from build123d import *

# Parameters (mm, degrees)
BASE_FLANGE2_DEPTH             = 1
EDGE_FLANGE1_STRIP_W           = 6
EDGE_FLANGE1_STRIP_H           = 1
EDGE_FLANGE1_STRIP_CUT_DEPTH   = 82.6
EDGE_FLANGE1_STRIP_2_W         = 6
EDGE_FLANGE1_STRIP_2_H         = 1
EDGE_FLANGE1_STRIP_CUT_2_DEPTH = 82.6
EDGE_FLANGE1_DEPTH             = 82.6
EDGE_FLANGE1_BEND_DEPTH        = 82.6
SKETCH16_W                     = 66.6
SKETCH16_H                     = 7
CUT_EXTRUDE1_DEPTH             = 138.553195479
FILLET1_R                      = 1
SKETCH17_R                     = 2
CUT_EXTRUDE2_DEPTH             = 138.553195479
FILLET2_R                      = 2.5


# Sheet-metal steps are written as plain solids
with BuildPart() as part:
    # Sketch1 → Base-Flange2 (new body)
    with BuildSketch(Plane(origin=(0, 0, 0), x_dir=(1, 0, 0), z_dir=(0, 1, 0))):
        Polygon((0, 0), (0, 82.6), (5, 82.6), (12.071067812, 89.671067812), (92.000932188, 89.671067812), (99.072, 82.6), (104.072, 82.6), (104.072, 0), (99.072, 0), (92.000932188, -7.071067812), (12.071067812, -7.071067812), (5, 0), align=None)
    extrude(amount=-BASE_FLANGE2_DEPTH)

    # Edge-Flange1 strip (across the edge) → Edge-Flange1 strip cut (cut)
    with BuildSketch(Plane(origin=(104.072, 0, 0), x_dir=(-1, 0, 0), z_dir=(0, 0, -1))):
        with Locations((-1, -0.5)):
            Rectangle(EDGE_FLANGE1_STRIP_W, EDGE_FLANGE1_STRIP_H)
    extrude(amount=EDGE_FLANGE1_STRIP_CUT_DEPTH, mode=Mode.SUBTRACT)

    # Edge-Flange1 strip 2 (across the edge) → Edge-Flange1 strip cut 2 (cut)
    with BuildSketch(Plane.XY.offset(-82.6)):
        with Locations((-1, -0.5)):
            Rectangle(EDGE_FLANGE1_STRIP_2_W, EDGE_FLANGE1_STRIP_2_H)
    extrude(amount=EDGE_FLANGE1_STRIP_CUT_2_DEPTH, mode=Mode.SUBTRACT)

    # Edge-Flange1 section (across the edge) → Edge-Flange1 (add)
    with BuildSketch(Plane(origin=(104.072, 0, 0), x_dir=(-1, 0, 0), z_dir=(0, 0, -1))):
        with BuildLine():
            Line((0, 1), (0, 7))
            Line((0, 7), (1, 7))
            Line((1, 7), (1, 1))
            ThreePointArc((1, 1), (1.292893219, 0.292893219), (2, 0))
            Line((2, 0), (2, -1))
            ThreePointArc((2, -1), (0.585786438, -0.414213562), (0, 1))
        make_face()
    extrude(amount=EDGE_FLANGE1_DEPTH)

    # Edge-Flange1 section 2 (across the edge) → Edge-Flange1 bend (add)
    with BuildSketch(Plane.XY.offset(-82.6)):
        with BuildLine():
            Line((0, 1), (0, 7))
            Line((0, 7), (1, 7))
            Line((1, 7), (1, 1))
            ThreePointArc((1, 1), (1.292893219, 0.292893219), (2, 0))
            Line((2, 0), (2, -1))
            ThreePointArc((2, -1), (0.585786438, -0.414213562), (0, 1))
        make_face()
    extrude(amount=EDGE_FLANGE1_BEND_DEPTH)

    # Sketch16 → Cut-Extrude1 (cut, through all)
    with BuildSketch(Plane(origin=(104.072, 0, 0), x_dir=(0, 0, -1), z_dir=(1, 0, 0))):
        with Locations((41.3, 4.5)):
            Rectangle(SKETCH16_W, SKETCH16_H)
    extrude(amount=-CUT_EXTRUDE1_DEPTH, mode=Mode.SUBTRACT)

    # Fillet1
    fillet1_edges = [part.edges().sort_by_distance(p)[0] for p in [
        (0.5, 7, -74.6),
        (0.5, 7, -8),
        (103.572, 7, -8),
        (103.572, 7, -74.6),
        (103.572, 7, 0),
        (103.572, 7, -82.6),
        (0.5, 7, -82.6),
        (0.5, 7, 0),
    ]]
    fillet(fillet1_edges, radius=FILLET1_R)

    # Sketch17 → Cut-Extrude2 (cut, through all)
    with BuildSketch(Plane(origin=(104.072, 0, 0), x_dir=(0, 0, -1), z_dir=(1, 0, 0))):
        with Locations(Location((4, 4, 0), (0, 0, 90))):
            Circle(SKETCH17_R)
        with Locations(Location((78.6, 4, 0), (0, 0, 90))):
            Circle(SKETCH17_R)
    extrude(amount=-CUT_EXTRUDE2_DEPTH, mode=Mode.SUBTRACT)

    # Fillet2
    fillet2_edges = [part.edges().sort_by_distance(p)[0] for p in [
        (12.071067812, -0.5, -89.671067812),
        (92.000932188, -0.5, -89.671067812),
        (92.000932188, -0.5, 7.071067812),
        (12.071067812, -0.5, 7.071067812),
    ]]
    fillet(fillet2_edges, radius=FILLET2_R)


solid = part.part
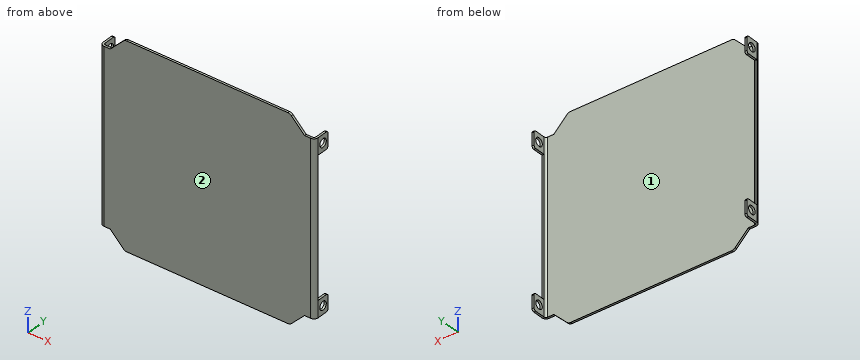
For this review, take the finished solid that the model builds, in its own axes (mm). Face numbers are marked on the shaded views. A direction names the side the tool comes from. Coordinates: 2 decimals unless noted, no trailing zeros. Write each loop counter-clockwise with the first axis right and the second up, starting at its lowest first coordinate (ties: lowest second). Pieces come first, ordered by that corner, then holes. Notation, with made-up numbers: (45.25, 5.5) -> (88.25, 5.5) arc R15 ccw to (88.25, 32.5) -> close; hole circle Ø8 at (-15.75, 79.5). An arc over 180 degrees is marked (long way). Write each question's results on one line, items separated by ' | '. Start each with the question number.
1) Wall thickness on L1, parallel to Z at x = 103.6, y = 4; L2, parallel to X at y = 3.75, z = -75.5; L3, parallel to Y at x = 99, z = -74.5: over which ranges is each line inside the solid? List them lowest first. Write a range as [from, to].
2) For the marked faces 1 and 2, list the 3-axis set-ups (+Z, -Z, +X, -X, +Y, -Y) from which the entire face can be reached by the end or side of a thin tool; tool diameter is ignored.
3) Consider section A-A (z = -4). Write out the cut boundary in (x, y), plus the area to 3 significant figures.
4) Consider section C-C (z = -42). Write out the cut boundary in (x, y).
5) Consider section B-B (y = 4). Give the number of separate pieces and of enclosed holes in the cut face, plus the area to 3 significant figures.
6) Consider section D-D (x = 74). Write out the cut boundary in (y, z).
7) Insertion check: pin 1 (0.8 mm diameter, centred on x = 0.5, z = -38, fed in from +Y); pin 2 (12 mm diameter, centred on x = 74.5, z = -27, fed in from +Y); pin 3 (0.5 mm diameter, centred on x = 0.5, y = 3.5, fed in from -Z); pin 4 (1.5 mm diameter, centred on x = 100.5, y = 1.5, fed in from +Z). Each pin has a flat end and moves straight along its axis. Give the tip position at first contact, or say it passes through.
Geometry says:
1) L1: [-82.6, -80.6], [-76.6, -74.6], [-8, -6], [-2, 0] | L2: [0, 1], [103.07, 104.07] | L3: [-1, 0]
2) face 1: +Z, -Z, +Y | face 2: +Z, -Z, +X, -X, -Y
3) outline: (0, 1) arc R2 ccw to (2, -1) -> (102.07, -1) arc R2 ccw to (104.07, 1) -> (104.07, 2) -> (103.07, 2) -> (103.07, 1) arc R1 cw to (102.07, 0) -> (2, 0) arc R1 cw to (1, 1) -> (1, 2) -> (0, 2) -> close; (0, 6) -> (1, 6) -> (1, 7) -> (0, 7) -> close; (103.07, 6) -> (104.07, 6) -> (104.07, 7) -> (103.07, 7) -> close | area: 109 mm^2
4) outline: (0, 1) arc R2 ccw to (2, -1) -> (102.07, -1) arc R2 ccw to (104.07, 1) -> (103.07, 1) arc R1 cw to (102.07, 0) -> (2, 0) arc R1 cw to (1, 1) -> close
5) separate pieces: 8 | enclosed holes: 0 | area: 16.0 mm^2
6) outline: (-1, -89.67) -> (0, -89.67) -> (0, 7.07) -> (-1, 7.07) -> close
7) pin 1: y = 1 | pin 2: y = 0 | pin 3: z = -82.6 | pin 4: through
